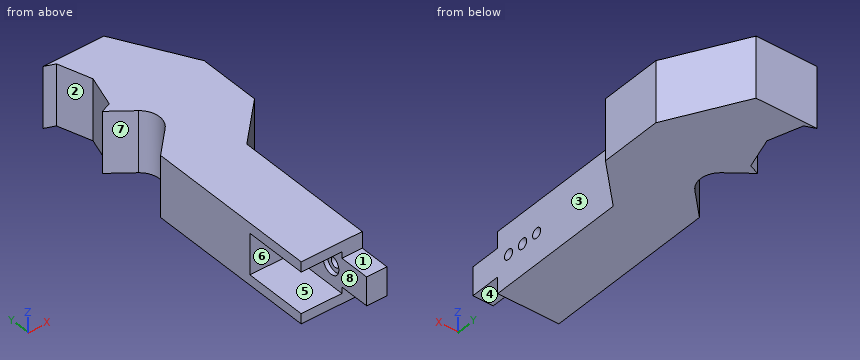
Autodesk Inventor part; units mm, degrees
ref_plane "YZ Plane" through (0, 0, 0) normal (1, 0, 0) x (0, 1, 0)
ref_plane "XZ Plane" through (0, 0, 0) normal (0, 1, 0) x (-1, 0, 0)
ref_plane "XY Plane" through (0, 0, 0) normal (0, 0, 1) x (1, 0, 0)
sketch "Sketch1" plane through (0, 0, 0) normal (0, 0, 1) x (1, 0, 0)
  line L0 (0, 0) -> (25, 0)
  line L1 (25, 0) -> (25, 40)
  line L2 (25, 40) -> (0, 40)
  line L3 (0, 40) -> (0, 0)
  dimension "d1" = 25
  dimension "d2" = 40
  dimension "d3" = 25
extrude "Extrusion1" add sketch "Sketch1" against normal blind 30
sketch "Sketch2" plane through (25, 0, 0) normal (1, 0, 0) x (0, 0, -1)
  line L0 (0, 0) -> (30, 0)
  circle A0 centre (15, 6.56) radius 2.46
extrude "Extrusion2" cut sketch "Sketch2" against normal blind 30
sketch "Sketch3" plane through (0, 0, 0) normal (-1, 0, 0) x (0, 0, 1)
  line L0 (0, 0) -> (-30, 0)
  line L1 (-25.05, 0) -> (-4.95, 0)
  line L2 (-4.95, 0) -> (-4.95, 33.12)
  line L3 (-4.95, 33.12) -> (-25.05, 33.12)
  line L4 (-25.05, 33.12) -> (-25.05, 0)
  dimension "d11" = 20.1
extrude "Extrusion3" cut sketch "Sketch3" against normal blind 20
sketch "Sketch4" plane through (0, 0, 0) normal (0, -1, 0) x (1, 0, 0)
  line L0 (20, -4.95) -> (20, -25.05)
  line L1 (20, -15) -> (25, -15)
  line L2 (25, 0) -> (25, -30)
  line L3 (20, -8.025) -> (25, -8.025)
  line L4 (25, -8.025) -> (25, -21.975)
  line L5 (25, -21.975) -> (20, -21.975)
  line L6 (20, -21.975) -> (20, -8.025)
  line L7 (20, -8.025) -> (25, -21.975) construction
  line L8 (25, -8.025) -> (20, -21.975) construction
  line L9 (25, -12.54) -> (25, -17.46)
  point P0 (0, 0)
  point P1 (22.5, -15)
  dimension "d14" = 13.95
extrude "Extrusion4" add sketch "Sketch4" along normal blind 15
sketch "Sketch5" plane through (20, 0, 0) normal (-1, 0, 0) x (0, 0, 1)
  circle A0 centre (-15, 6.56) radius 2.46
  circle A1 centre (-15, 6.56) radius 4.7025
  circle A2 centre (-15, 6.56) radius 2.46
  circle A3 centre (-15, 6.56) radius 2.46
  point P0 (0, 0)
  dimension "d17" = 9.405
extrude "Extrusion5" cut sketch "Sketch5" against normal blind 2.1
sketch "Sketch6" plane through (25, 0, 0) normal (1, 0, 0) x (0, 0, -1)
  circle A0 centre (15, 6.56) radius 4.7025
  line L0 (15, 6.56) -> (15, 23.56)
  circle A1 centre (15, 23.56) radius 2.46
  point P0 (0, 0)
  dimension "d20" = 17
  dimension "d21" = 4.92
extrude "Extrusion6" cut sketch "Sketch6" against normal blind 10 contours A1
sketch "Sketch7" plane through (20, 0, 0) normal (-1, 0, 0) x (0, 0, 1)
  circle A0 centre (-15, 23.56) radius 2.46
  circle A1 centre (-15, 23.56) radius 4.7025
  point P0 (0, 0)
  dimension "d24" = 9.405
extrude "Extrusion7" cut sketch "Sketch7" against normal blind 2.1
sketch "Sketch9" plane through (25, 0, 0) normal (1, 0, 0) x (0, 0, -1)
  circle A0 centre (15, 6.56) radius 2.46
  circle A1 centre (15, 6.56) radius 2.46
  circle A2 centre (15, 23.56) radius 2.46
  circle A3 centre (15, 23.56) radius 2.46
  line L0 (30, 40) -> (30, 0)
  line L1 (30, 0) -> (30, 40)
  line L2 (30, 40) -> (0, 40)
  line L3 (0, 40) -> (0, 0)
  line L4 (0, 0) -> (8.025, 0)
  line L5 (21.975, 0) -> (21.975, -15)
  line L6 (21.975, -15) -> (8.025, -15)
  line L7 (8.025, -15) -> (8.025, 0)
  line L8 (0, 0) -> (8.025, 0)
  line L9 (21.975, 0) -> (30, 0)
extrude "Extrusion8" add sketch "Sketch9" along normal blind 5
sketch "Sketch10" plane through (0, 40, 0) normal (0, 1, 0) x (1, 0, 0)
  line L0 (0, 30) -> (30, 30)
  line L1 (30, 0) -> (0, 0)
  line L2 (0, 30) -> (30, 30)
  line L3 (30, 30) -> (30, 0)
  line L4 (30, 0) -> (0, 0)
  line L5 (0, 0) -> (0, 30)
extrude "Extrusion9" add sketch "Sketch10" along normal blind 30
sketch "Sketch12" plane through (30, 0, 0) normal (1, 0, 0) x (0, 0, -1)
  circle A0 centre (15, 6.56) radius 2.46
  line L0 (15, 6.56) -> (15, 15.06)
  circle A1 centre (15, 15.06) radius 2.525
  point P0 (0, 0)
  dimension "d31" = 8.5
  dimension "d33" = 5.05
extrude "Extrusion10" cut sketch "Sketch12" against normal blind 30 contours A1
sketch "Sketch15" plane through (0, 0, -25.05) normal (-1, 0, 0) x (0, 0, 1)
  line L0 (0, 33.12) -> (20.1, 33.12)
  line L1 (20.1, 33.12) -> (20.1, 0)
  line L2 (0, 33.12) -> (20.1, 33.12)
  line L3 (20.1, 33.12) -> (20.1, 31.1)
  line L4 (20.1, 31.1) -> (0, 31.1)
  line L5 (0, 31.1) -> (0, 33.12)
  point P0 (25.05, 0)
  dimension "d57" = 2.02
extrude "Extrusion13" add sketch "Sketch15" against normal blind 20
sketch "Sketch17" plane through (0, 0, 0) normal (0, 0, 1) x (1, 0, 0)
  line L0 (0, 70) -> (30, 70)
  line L1 (30, 70) -> (50.0622, 90.0622)
  line L2 (30, 70) -> (80, 70) construction
  line L3 (11.9522, 97.2454) -> (0, 85.2932)
  line L4 (0, 70) -> (0, 85.2932)
  line L5 (0, 70) -> (0, 0)
  line L6 (0, 70) -> (30, 70)
  line L7 (10.923, 112.2849) -> (0, 120.567)
  line L8 (50.0622, 105.3553) -> (50.0622, 120.567)
  line L9 (50.0622, 105.3553) -> (50.0622, 90.0622)
  arc A0 (11.9522, 97.2454) -> (10.923, 112.2849) centre (4.8811, 104.3165) ccw
  line L10 (0, 156.567) -> (30, 156.567)
  line L11 (30, 156.567) -> (50.0622, 120.567)
  line L12 (5, 154.567) -> (0, 156.567)
  line L13 (5, 122.567) -> (0, 120.567)
  line L14 (5, 122.567) -> (10, 138.567)
  line L15 (10, 138.567) -> (5, 154.567)
  dimension "d61" = 45
  dimension "d62" = 32.0271
  dimension "d72" = 10
extrude "Extrusion14" add sketch "Sketch17" against normal blind 30
properties part number "rec_c_32mm_x_30mm"
Input: part model. Units: mm. Frame: model coordinates. Face numbers are marked on the shaded views. A direction names the side the tool comes from. Round coordinates to 2 decimals unless told otherwise and drop trailing zeros. Loops run counter-clockwise (first coordinate to the right, second up) from the corner with the lowest first, then second, coordinate; pieces in that order, holes last. Notation, with made-up numbers: (22, 24.5) - (71, 24.5) arc R17 cw to (71, 38.5) - close; hole circle Ø8 at (-18.75, -14). An arc over 180 degrees is marked (long way). One line per item, written item: value. Start each with the question number.
(1) Ray query, line 1 (Y direction, x = 21.15, z = -15) (1 decimal); line 2 (Y direction, x = 24, z = -15) (3 decimals); line 3 (Z direction, x = 21, y = 6). Return the intervals inside material, ascending. Write a range as [from, to].
(2) Section A-A, the plane y = 23.56. Return loops of the section in (x, z).
(3) Access query for the marked faces 1, 2, 3, 4 and 5. Directions: +Z, -Z, +X, -X, +Y, -Y. A direction counts if a zero-diameter tool reaches every point of the face in a straight line with its end or side. Return the directions, or none.
(4) Section D-D, the plane x = 36. Return loops of the section in (y, z), plus the area to 3 significant figures.
(5) Section B-B, the plane z = -15. Count the separate pieces of the cut face and the enclosed holes in it, plus the area to 3 significant figures.
(6) Contact query for flat-ended pins moving along their axis: P1, Ø6.5, axis at x = 13.5, z = -3.5, coming from the -Y side; P2, Ø6, axis at y = 9.5, z = -13, coming from the -X side; P3, Ø1.5, axis at x = 7, y = 19, coming from the +Z side; P4, Ø5.5, axis at y = 23.56, z = -15, coming from the -X side. Output: stop coordinate, or through.
(7) Draft query along Y for the marked faces 6, 7 and 8. Return one class per face: +Y half, -Y half, draft (parallel to the pull), parting line (faces both ways), or undercut.
(8) Section C-C, the plane y = 45. Return loops of the section in (x, z), plus the area to 3 significant figures.
Results below:
1. line 1: [-15, 1.9], [11.3, 12.5], [17.6, 18.9], [28.3, 156.6]
1. line 2: [-15, 4.1], [9.02, 12.535], [17.585, 21.1], [26.02, 156.567]
1. line 3: [-30, -19.67], [-10.33, 0]
2. outline: (0, -30) - (30, -30) - (30, -17.46) - (22.1, -17.46) - (22.1, -19.7) - (20, -19.7) - (20, -25.05) - (0, -25.05) - close; (0, -4.95) - (20, -4.95) - (20, -10.3) - (22.1, -10.3) - (22.1, -12.54) - (30, -12.54) - (30, 0) - (0, 0) - close
3. face 1: +Z, +X, -X, -Y
3. face 2: +Z, -Z, -X
3. face 3: +Z, -Z, +X, -Y
3. face 4: -Z, +X, -X, -Y
3. face 5: -X, -Y
4. outline: (76, -30) - (145.8, -30) - (145.8, 0) - (76, 0) - close
4. area: 2,090 mm^2
5. separate pieces: 4
5. enclosed holes: 0
5. area: 4,660 mm^2
6. P1: y = 0
6. P2: x = 20
6. P3: z = 0
6. P4: x = 22.1
7. face 6: -Y half
7. face 7: undercut
7. face 8: draft
8. outline: (0, -30) - (30, -30) - (30, 0) - (0, 0) - close
8. area: 900 mm^2
